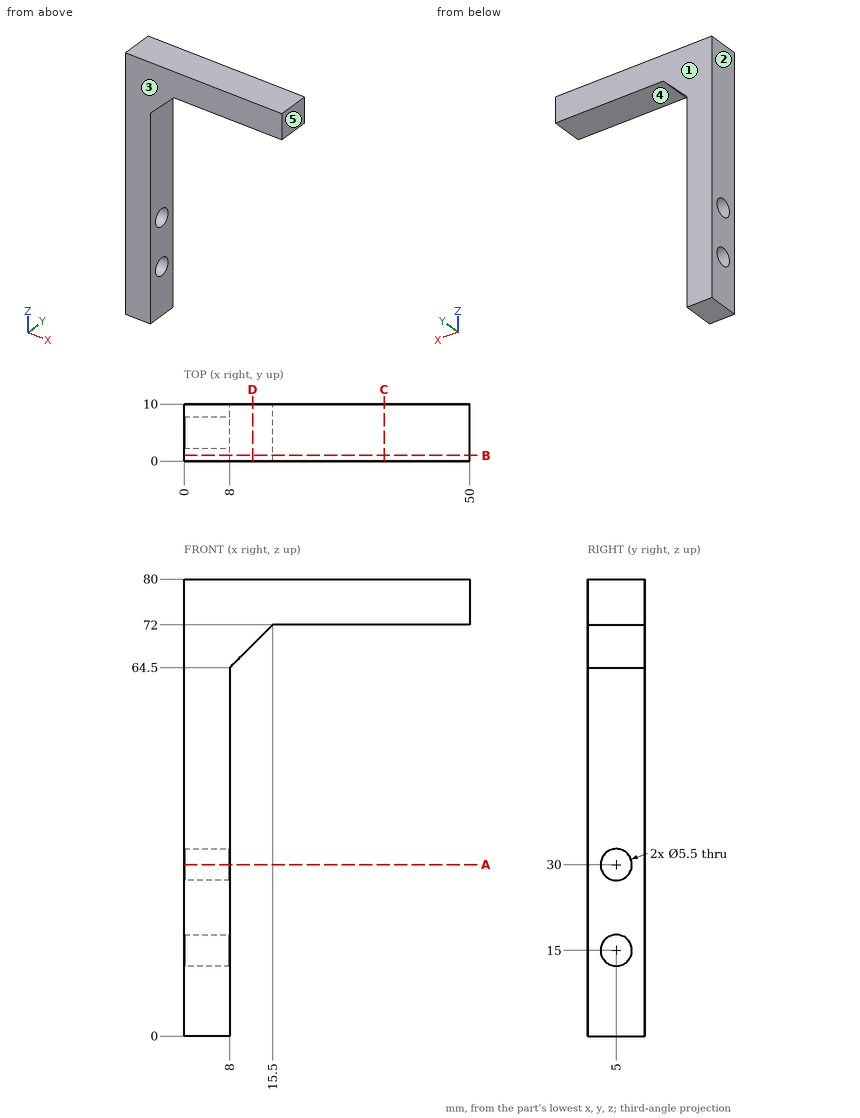
Geometry: see drawing. Coordinates: mm, zero at the bounding-box minimum. A direction names the side the tool comes from. Coordinates: 2 decimals unless noted, no trailing zeros. Write each loop counter-clockwise with the first axis right and the second up, starting at its lowest first coordinate (ties: lowest second). Pieces come first, ordered by that corner, then holes. Notation, with made-up numbers: (-10.5, 56.5) - (30.5, 56.5) arc R25 ccw to (30.5, 94.5) - close; hole circle Ø6 at (19.25, 23.25). An arc over 180 degrees is marked (long way). Put each result on its own line as item: value. Start each with the question number.
1) Cut plane D-D (x = 12). Return the cut outline in (y, z), plus the area to 3 significant figures.
2) Cut plane A-A (z = 30). Return the cut outline in (x, y), plus the area to 3 significant figures.
3) Contact query for a flat-ended pin moving along its axis: pin 1 (8 mm diameter, centred on x = 42.5, z = 71.5, fed in from -Y). Output: stop coordinate, or through.
4) Ray query, L1, parallel to Y at x = 3, z = 30; L2, parallel to X at y = 1.5, z = 29.5; L3, parallel to Z at x = 31, y = 6.25. Return the intervals inside material, ascending.
5) Cut plane B-B (y = 1). Return the cut outline in (x, z).
6) Cut plane C-C (x = 35). Return the cut outline in (y, z), plus the area to 3 significant figures.
7) Reachability of the marked faces 4 and 5 from +Z, -Z, +X, -X, +Y, -Y: full face, straight path, thin tool, end or side. Return the list, or none.
8) Mould query, pull axis Y, two halves, no side actions, for the marked faces 1, 2 and 3. Classes: pulls with the +Y half, pulls with the -Y half, needs draft (parallel to the pull), parting line crosses it, or undercut.
Resolved:
1. outline: (0, 68.5) - (10, 68.5) - (10, 80) - (0, 80) - close
1. area: 115 mm2
2. outline: (0, 0) - (8, 0) - (8, 2.25) - (0, 2.25) - close; (0, 7.75) - (8, 7.75) - (8, 10) - (0, 10) - close
2. area: 36.0 mm2
3. pin 1: stops at y = 0
4. L1: y = 0 to 2.25, 7.75 to 10
4. L2: x = 0 to 8
4. L3: z = 72 to 80
5. outline: (0, 0) - (8, 0) - (8, 64.5) - (15.5, 72) - (50, 72) - (50, 80) - (0, 80) - close
6. outline: (0, 72) - (10, 72) - (10, 80) - (0, 80) - close
6. area: 80.0 mm2
7. face 4: -Z, +X, +Y, -Y
7. face 5: +Z, -Z, +X, +Y, -Y
8. face 1: pulls with the +Y half
8. face 2: needs draft
8. face 3: pulls with the -Y half
